```python
from build123d import *

# Parameters (mm, degrees)
CHAMFER_1_SIZE      = 0.16
CHAMFER_2_SIZE      = 0.14
CUT_EXTRUDE_1_DEPTH = 2
CUT_EXTRUDE_2_REACH = 16.849
SKETCH_4_R          = 0.75


with BuildPart() as part:
    # 草图2 → 旋转1 (revolve)
    with BuildSketch(Plane.XY):
        Polygon((-1.5, 0), (-1.5, -2), (0, -2.866025404), (0, -14), (-2, -14), (-2, -4), (-3.5, -4), (-3.5, 0), align=None)
    revolve(axis=Axis((0, -2.866025404, 0), (0, -1, 0)))

    # 倒角1
    chamfer_1_edges = [part.edges().sort_by_distance(p)[0] for p in [
        (2, -14, 0),
    ]]
    chamfer(chamfer_1_edges, length=CHAMFER_1_SIZE)

    # 倒角2
    chamfer_2_edges = [part.edges().sort_by_distance(p)[0] for p in [
        (3.5, 0, 0),
    ]]
    chamfer(chamfer_2_edges, length=CHAMFER_2_SIZE)

    # 草图3 → 切除-拉伸1 (cut)
    with BuildSketch(Plane(origin=(0, 0, 0), x_dir=(-1, 0, 0), z_dir=(0, 1, 0))):
        Polygon((-0.866025404, 1.5), (-1.732050808, 0), (-0.866025404, -1.5), (0.866025404, -1.5), (1.732050808, 0), (0.866025404, 1.5), align=None)
    extrude(amount=-CUT_EXTRUDE_1_DEPTH, mode=Mode.SUBTRACT)

    # 切除-拉伸2: up to this cone (the profile starts outside it)
    cut_extrude_2_end = Plane(origin=(0, -14, 0), z_dir=(0, 1, 0)).offset(11.133975596) * Cone(1.732e-06, 10.76473977, 6.215024404, align=(Align.CENTER, Align.CENTER, Align.MIN), mode=Mode.PRIVATE)
    # 草图4 → 切除-拉伸2 (cut, up to the surface)
    with BuildSketch(Plane.XZ.offset(14), mode=Mode.PRIVATE) as cut_extrude_2_sk1:
        Circle(SKETCH_4_R)
    cut_extrude_2_tool1 = extrude(cut_extrude_2_sk1.sketch, amount=-CUT_EXTRUDE_2_REACH, mode=Mode.PRIVATE) - cut_extrude_2_end
    add(cut_extrude_2_tool1.solids().sort_by_distance((0, -14, 0))[0], mode=Mode.SUBTRACT)


solid = part.part
```
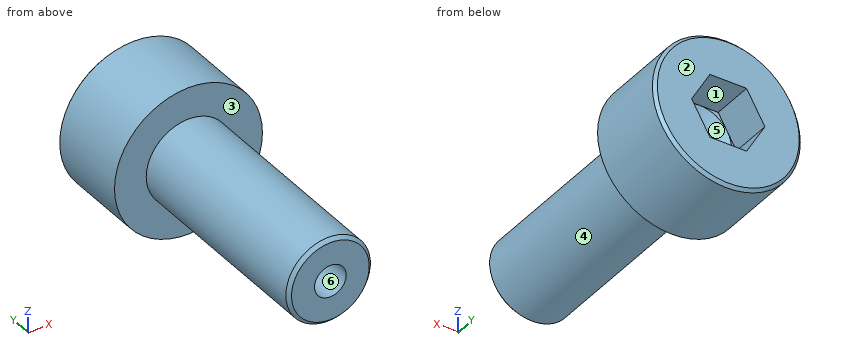
Could you check a few things on this model? Use its own coordinates, in mm. Face numbers are marked on the shaded views. A direction names the side the tool comes from. Give positions to 0.01 mm unless a question says otherwise; leave off trailing zeros. Write each loop counter-clockwise with the first axis right and the second up, starting at its lowest first coordinate (ties: lowest second). Pieces come first, ordered by that corner, then holes. Notation, with made-up numbers: (54.5, -6) -> (96.5, -6) arc R24 ccw to (96.5, 4) -> close; hole circle Ø1 at (16, 37). An arc over 180 degrees is marked (long way). Write each question's results on one line, items separated by ' | '.
1. On a 3-axis mill with a long thin cutter (end or side, diameter ignored), from which of +Z, -Z, +X, -X, +Y, -Y can I reach the whole of each face in a straight line? I mean the marked faces 1 and 2. Say none if no direction works.
Check sheet entries:
face 1: +Y | face 2: +Z, -Z, +X, -X, +Y
2. If we mould it in two halves opening along Z, with no side actions, what happens to the marked faces 3, 4, 5 and 6? For each: released by +Z, released by -Z, zero draft, split by the parting line, or undercut.
Check sheet entries:
face 3: zero draft | face 4: split by the parting line | face 5: undercut | face 6: undercut
3. Will these pins go through, and if not, where does the flat tip stop? pin 1 Ø1.2 at (x, z) = (0, 0) entering from -Y; pin 2 Ø1 at (x, z) = (-2.5, -1) entering from -Y; pin 3 Ø1 at (x, y) = (1.5, -7.5) entering from +Z; pin 4 Ø1.5 at (y, z) = (-12.5, 1) entering from -X.
Check sheet entries:
pin 1: passes through | pin 2: stops at y = -4 | pin 3: stops at z = 1.73 | pin 4: stops at x = -1.98
4. I need wall thicknesses on L1, parallel to Z at x = 0, y = -5.75; L2, parallel to Y at x = 2, z = 1.5; L3, parallel to Y at x = 0.25, z = 0.75. Which ranges of each line are inside material? Lowest first, please.
Check sheet entries:
L1: z = -2 to -0.75, 0.75 to 2 | L2: y = -4 to 0 | L3: y = -14 to -2.41
5. I want a section at A-A, the plane y = -3.75. Write out the boundary of the cut face in (x, z).
Check sheet entries:
outline: circle Ø7 at (0, 0); hole circle Ø1.5 at (0, 0)
